Check sheet for the drawn part. Datum: minimum x, y, z corner. Units: mm. Round coordinates to 2 decimals unless told otherwise and drop trailing zeros. Loops run counter-clockwise (first coordinate to the right, second up) from the corner with the lowest first, then second, coordinate; pieces in that order, holes last. Notation, with made-up numbers: (26, -27) -> (42, -27) arc R20 ccw to (42, -15) -> close; hole circle Ø3 at (40, -11). An arc over 180 degrees is marked (long way). Use CSV: the item, a comma, the result in double quotes. Start each with the question number.
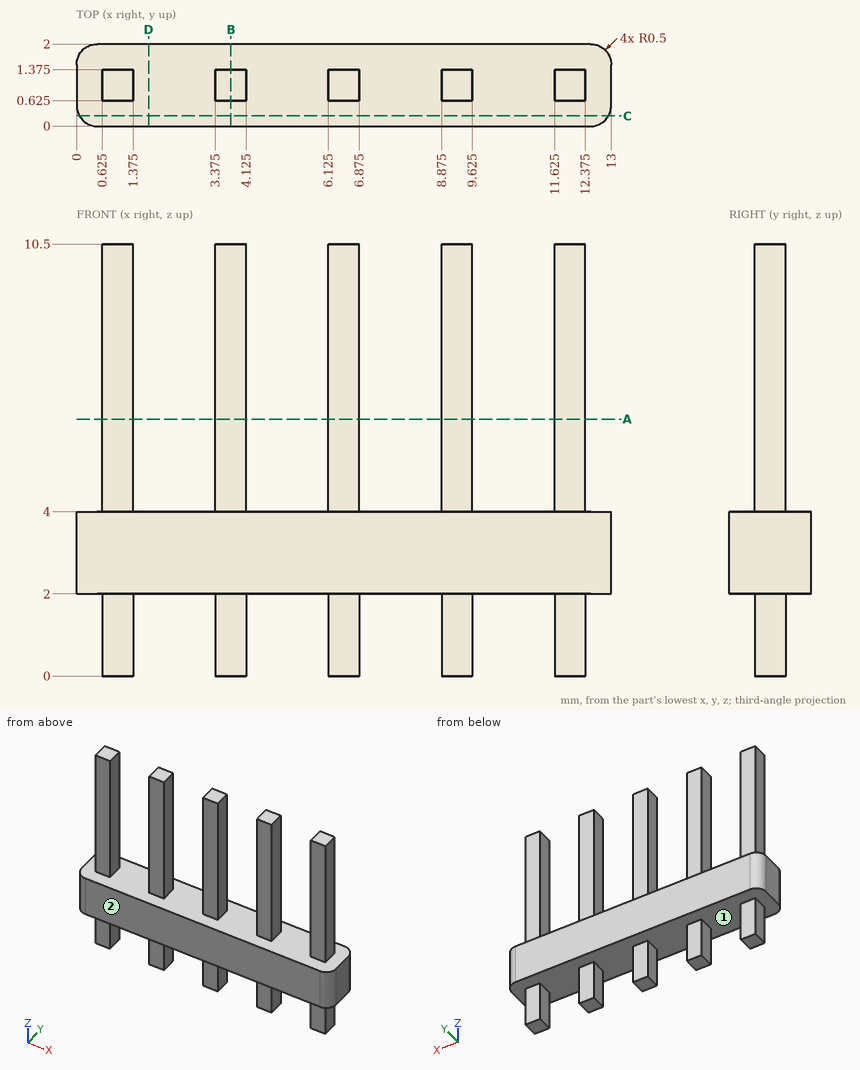
Q1. Cross-section at B-B (x = 3.75). Record the boundary of the cut face in (y, z) (3 decimals).
Q2. Cross-section at C-C (y = 0.25). Record the boundary of the cut face in (x, z), and give its area (3 significant figures).
Q3. Cross-section at A-A (z = 6.25). Record the boundary of the cut face in (x, y) (3 decimals).
Q4. Thickness scan on L1, parallel to X at y = 0.95, z = 9 (3 decimals); L2, parallel to Z at x = 5, y = 0.1; L3, parallel to Y at x = 3.5, z = 5.75 (3 decimals). Record the ranges inside material, lowest first. Write a range as from..to.
Q5. Depth check by flat-ended pin: pin 1 Ø5 at (x, z) = (11, 4.5) entering from -Y; pin 2 Ø1.5 at (x, z) = (5.5, 5.5) entering from -Y (3 decimals); pin 3 Ø0.8 at (y, z) = (1, 1) entering from +X (3 decimals); pin 4 Ø0.6 at (y, z) = (1, 7.5) entering from -X (3 decimals). Enter the tip coordinate at first touch or a pass-through.
Q6. Cross-section at D-D (x = 1.75). Record the boundary of the cut face in (y, z).
Q7. Release check for a two-part mould opening along X. For the marked faces 1 and 2 record: +X half, -X half, draft (parallel to the pull), parting line (faces both ways), or undercut.
Answer list:
1,outline,"(0, 2) -> (0.625, 2) -> (0.625, 0) -> (1.375, 0) -> (1.375, 2) -> (2, 2) -> (2, 4) -> (1.375, 4) -> (1.375, 10.5) -> (0.625, 10.5) -> (0.625, 4) -> (0, 4) -> close"
2,outline,"(0.07, 2) -> (12.93, 2) -> (12.93, 4) -> (0.07, 4) -> close"
2,area,"25.7 mm2"
3,outline,"(0.625, 0.625) -> (1.375, 0.625) -> (1.375, 1.375) -> (0.625, 1.375) -> close; (3.375, 0.625) -> (4.125, 0.625) -> (4.125, 1.375) -> (3.375, 1.375) -> close; (6.125, 0.625) -> (6.875, 0.625) -> (6.875, 1.375) -> (6.125, 1.375) -> close; (8.875, 0.625) -> (9.625, 0.625) -> (9.625, 1.375) -> (8.875, 1.375) -> close; (11.625, 0.625) -> (12.375, 0.625) -> (12.375, 1.375) -> (11.625, 1.375) -> close"
4,L1,"x = 0.625..1.375, 3.375..4.125, 6.125..6.875, 8.875..9.625, 11.625..12.375"
4,L2,"z = 2..4"
4,L3,"y = 0.625..1.375"
5,pin 1,"stops at y = 0"
5,pin 2,"stops at y = 0.625"
5,pin 3,"stops at x = 12.375"
5,pin 4,"stops at x = 0.625"
6,outline,"(0, 2) -> (2, 2) -> (2, 4) -> (0, 4) -> close"
7,face 1,"undercut"
7,face 2,"draft"
